Could you check a few things on this drawing? It's one solid part, dimensions in mm from its lowest x, y, z. A direction names the side the tool comes from. Give positions to 0.01 mm unless a question says otherwise; leave off trailing zeros. Loops run counter-clockwise (first coordinate to the right, second up) from the corner with the lowest first, then second, coordinate; pieces in that order, holes last. Notation, with made-up numbers: M -12.5,-38.75 L 33.5,-38.75 A25 ccw 33.5,-4.75 Z; hole C 82,-36.75 d8. An arc over 180 degrees is marked long. Write each question's results on one line, items separated by ' | '. Start each with the question number.
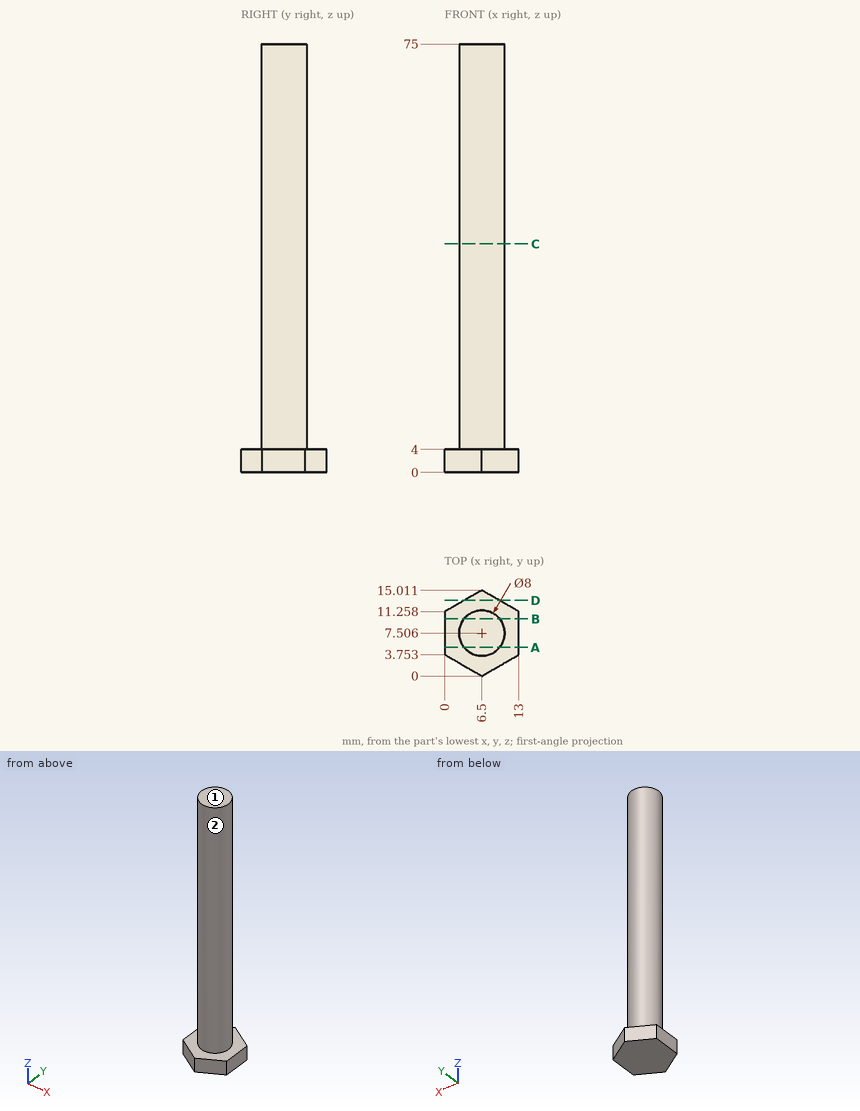
1) If we section it at D-D on y = 13.25: Write out the boundary of the cut face in (x, z), plus the area to 3 significant figures.
2) If we section it at B-B on y = 10: Write out the boundary of the cut face in (x, z), plus the area to 3 significant figures.
3) I'm going to push flat-ended pins straight in: P1, Ø4, axis at y = 4.5, z = 31.5, coming from the -X side; P2, Ø6, axis at y = 6, z = 23.5, coming from the -X side; P3, Ø1, axis at y = 9.5, z = 44.5, coming from the +X side. Where does each tip first touch, or does it pass through?
4) Which directions (+Z, -Z, +X, -X, +Y, -Y) give clear straight access to the entire face, cutting with the end or side of a thin tool? Please do the marked faces 1 and 2.
5) If we section it at A-A on y = 5: Write out the boundary of the cut face in (x, z), plus the area to 3 significant figures.
6) Please list where these lines run through material, in increasing order: line 1 (Z direction, x = 12.25, y = 6.75); line 2 (X direction, y = 7.25, z = 10); line 3 (Y direction, x = 8.75, z = 29). Write a range as from..to.
7) If we section it at C-C on z = 40: Write out the boundary of the cut face in (x, y) (1 decimal).
Calculated:
1) outline: M 3.45,0 L 9.55,0 L 9.55,4 L 3.45,4 Z | area: 24.4 mm2
2) outline: M 0,0 L 13,0 L 13,4 L 9.63,4 L 9.63,75 L 3.37,75 L 3.37,4 L 0,4 Z | area: 496 mm2
3) P1: stops at x = 2.63 | P2: stops at x = 2.5 | P3: stops at x = 10.21
4) face 1: +Z, +X, -X, +Y, -Y | face 2: +Z
5) outline: M 0,0 L 13,0 L 13,4 L 9.62,4 L 9.62,75 L 3.38,75 L 3.38,4 L 0,4 Z | area: 495 mm2
6) line 1: z = 0..4 | line 2: x = 2.51..10.49 | line 3: y = 4.2..10.81
7) outline: C 6.5,7.5 d8
